Model file for the job. Use its own axes, mm. Face numbers are marked on the shaded views. A direction names the side the tool comes from. Coordinates: 2 decimals unless noted, no trailing zeros. Write each loop counter-clockwise with the first axis right and the second up, starting at its lowest first coordinate (ties: lowest second). Pieces come first, ordered by that corner, then holes. Notation, with made-up numbers: M 44.5,-29.5 L 53.5,-29.5 A24 ccw 53.5,-1.5 Z; hole C 61,86 d2. An arc over 180 degrees is marked long. One line per question, with ' | ' between items. Start each with the question number.
(1) Cut at B-B (x = 35). Write the cut outline in (y, z).
(2) Cut at A-A (y = -3). Write the cut outline in (x, z).
(3) Tool access for the marked faces 1 and 2: list every direction of +Z, -Z, +X, -X, +Y, -Y with a clear straight run to the whole face (end or side of a thin tool).
(4) Cut at C-C (x = 45). Write the cut outline in (y, z).
(5) Cut at D-D (z = -12). Write the cut outline in (x, y).
(6) Wall check: probe 1 along X at (y, z) = (-4.75, 12); probe 2 along X at (y, z) = (-7.6, 12); probe 3 along Z at (x, y) = (15, -7.9). Give the ranges that are in metal, low to high.
(7) Flat gauge pins, fed straight in: pin 1 Ø3 at (y, z) = (-7.5, 1) entering from -X; pin 2 Ø3 at (x, z) = (69, 12) entering from -Y; pin 3 Ø1.5 at (x, y) = (23, -8) entering from -Z; pin 4 Ø1.5 at (x, z) = (66, -3) entering from +Y. Where does each tip first touch, or does it go through?
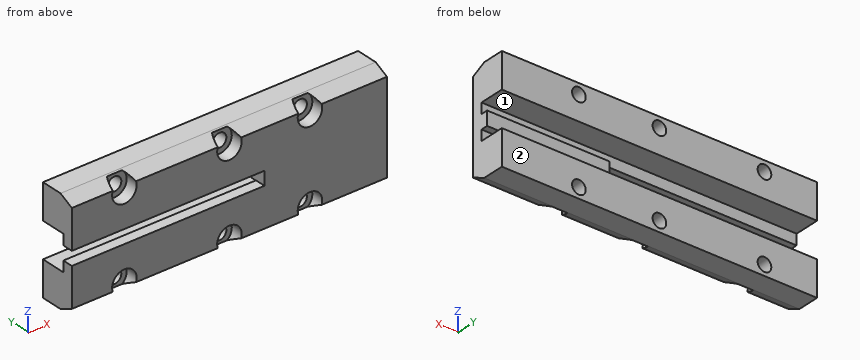
from build123d import *

# Parameters (mm, degrees)
EXTRUDE_1_DEPTH     = 90
EXTRUDE_1_2_DEPTH   = 90
SKETCH_3_R          = 1.95
CUT_EXTRUDE_1_DEPTH = 92.809803398
SKETCH_5_W          = 35
SKETCH_5_H          = 5
EXTRUDE_2_DEPTH     = 2
SKETCH_7_R          = 3.5
CUT_EXTRUDE_2_DEPTH = 3.5


with BuildPart() as part:
    # Sketch 1 → Extrude 1 (new body)
    with BuildSketch(Plane(origin=(0, 0, 0), x_dir=(0, 0, -1), z_dir=(1, 0, 0))):
        Polygon((-15, 0), (-15, -6.2), (-13.081136552, -10.2), (-1.95, -10.2), (-1.95, -7.2), (-5, -7.2), (-5, 0), align=None)
    extrude(amount=EXTRUDE_1_DEPTH)


with BuildPart() as body_2:
    # Sketch 1 → Extrude 1 2 (new body)
    with BuildSketch(Plane(origin=(0, 0, 0), x_dir=(0, 0, -1), z_dir=(1, 0, 0))):
        Polygon((13.081136552, -10.2), (15, -6.2), (15, 0), (5, 0), (5, -7.2), (1.95, -7.2), (1.95, -10.2), align=None)
    extrude(amount=EXTRUDE_1_2_DEPTH)


with BuildPart() as cut_extrude_1_tool:
    # Sketch 3 → Cut-Extrude 1 (new, through all)
    with BuildSketch(Plane.XZ.offset(10.2)):
        with Locations(Location((15, 12, 0), (0, 0, 270))):
            Circle(SKETCH_3_R)
        with Locations(Location((45, 12, 0), (0, 0, 270))):
            Circle(SKETCH_3_R)
        with Locations(Location((68, 12, 0), (0, 0, 270))):
            Circle(SKETCH_3_R)
        with Locations(Location((68, -12, 0), (0, 0, 270))):
            Circle(SKETCH_3_R)
        with Locations(Location((45, -12, 0), (0, 0, 270))):
            Circle(SKETCH_3_R)
        with Locations(Location((15, -12, 0), (0, 0, 270))):
            Circle(SKETCH_3_R)
    extrude(amount=-CUT_EXTRUDE_1_DEPTH)


with BuildPart() as part_1:
    add(part.part)

    # Cut-Extrude 1: cut by cut_extrude_1_tool
    add(cut_extrude_1_tool.part, mode=Mode.SUBTRACT)



with BuildPart() as body_2_1:
    add(body_2.part)

    # Cut-Extrude 1: cut by cut_extrude_1_tool
    add(cut_extrude_1_tool.part, mode=Mode.SUBTRACT)


with BuildPart() as part_2:
    add(part_1.part)

    add(body_2_1.part)  # Extrude 2 merges body 2
    # Sketch 5 → Extrude 2 (add, symmetric)
    with BuildSketch(Plane.XY):
        with Locations((72.5, -7.7)):
            Rectangle(SKETCH_5_W, SKETCH_5_H)
    extrude(amount=EXTRUDE_2_DEPTH, both=True)

    # Sketch 7 → Cut-Extrude 2 (cut)
    with BuildSketch(Plane.XZ.offset(10.2)):
        with Locations((15, -12)):
            Circle(SKETCH_7_R)
        with Locations((45, -12)):
            Circle(SKETCH_7_R)
        with Locations((68, -12)):
            Circle(SKETCH_7_R)
        with Locations((45, 12)):
            Circle(SKETCH_7_R)
        with Locations((68, 12)):
            Circle(SKETCH_7_R)
        with Locations((15, 12)):
            Circle(SKETCH_7_R)
    extrude(amount=-CUT_EXTRUDE_2_DEPTH, mode=Mode.SUBTRACT)


solid = part_2.part
Filled in:
1) outline: M -10.2,-13.08 L -6.2,-15 L 0,-15 L 0,-5 L -7.2,-5 L -7.2,-1.95 L -10.2,-1.95 Z; M -10.2,1.95 L -7.2,1.95 L -7.2,5 L 0,5 L 0,15 L -6.2,15 L -10.2,13.08 Z
2) outline: M 0,-15 L 90,-15 L 90,-5 L 0,-5 Z; M 0,5 L 90,5 L 90,15 L 0,15 Z; hole C 15,-12 d3.9; hole C 15,12 d3.9; hole C 45,-12 d3.9; hole C 45,12 d3.9; hole C 68,-12 d3.9; hole C 68,12 d3.9
3) face 1: +X, -X, +Y | face 2: +Z, -Z, +X, -X, +Y
4) outline: M -10.2,-8.5 L -6.7,-8.5 L -6.7,-10.05 L 0,-10.05 L 0,-5 L -7.2,-5 L -7.2,-1.95 L -10.2,-1.95 Z; M -10.2,1.95 L -7.2,1.95 L -7.2,5 L 0,5 L 0,10.05 L -6.7,10.05 L -6.7,8.5 L -10.2,8.5 Z; M -6.7,-14.76 L -6.2,-15 L 0,-15 L 0,-13.95 L -6.7,-13.95 Z; M -6.7,13.95 L 0,13.95 L 0,15 L -6.2,15 L -6.7,14.76 Z
5) outline: M 0,-10.2 L 11.5,-10.2 L 11.5,-6.7 L 13.05,-6.7 L 13.05,0 L 0,0 Z; M 16.95,-6.7 L 18.5,-6.7 L 18.5,-10.2 L 41.5,-10.2 L 41.5,-6.7 L 43.05,-6.7 L 43.05,0 L 16.95,0 Z; M 46.95,-6.7 L 48.5,-6.7 L 48.5,-10.2 L 64.5,-10.2 L 64.5,-6.7 L 66.05,-6.7 L 66.05,0 L 46.95,0 Z; M 69.95,-6.7 L 71.5,-6.7 L 71.5,-10.2 L 90,-10.2 L 90,0 L 69.95,0 Z
6) probe 1: 0 to 13.05, 16.95 to 43.05, 46.95 to 66.05, 69.95 to 90 | probe 2: 0 to 11.5, 18.5 to 41.5, 48.5 to 64.5, 71.5 to 90 | probe 3: -8.5 to -1.95, 1.95 to 8.5
7) pin 1: x = 0 | pin 2: y = -6.7 | pin 3: z = -14.5 | pin 4: y = -7.2
